```python
from build123d import *

# Parameters (mm, degrees)
SKETCH_1_W          = 60
SKETCH_1_H          = 95
EXTRUDE_1_DEPTH     = 5
SKETCH_2_R          = 1.5
SKETCH_2_R_2        = 1.25
CUT_EXTRUDE_1_DEPTH = 5
FILLET_1_R          = 5
CUT_EXTRUDE_4_DEPTH = 5
FILLET_4_R          = 0.5
FILLET_5_R          = 0.5


with BuildPart() as part:
    # 草图1 → 凸台-拉伸1 (new body)
    with BuildSketch(Plane(origin=(0, 0, 0), x_dir=(1, 0, 0), z_dir=(0, 1, 0))):
        Rectangle(SKETCH_1_W, SKETCH_1_H)
    extrude(amount=EXTRUDE_1_DEPTH)

    # 草图2 → 切除-拉伸1 (cut)
    with BuildSketch(Plane(origin=(0, 5, 0), x_dir=(1, 0, 0), z_dir=(0, 1, 0))):
        with Locations(Location((-24.605, 43.54, 0), (0, 0, 270))):
            Circle(SKETCH_2_R)
        with Locations(Location((24.605, 43.54, 0), (0, 0, 90))):
            Circle(SKETCH_2_R)
        with Locations(Location((24.605, -43.54, 0), (0, 0, 270))):
            Circle(SKETCH_2_R)
        with Locations(Location((-24.605, -43.54, 0), (0, 0, 90))):
            Circle(SKETCH_2_R)
        with Locations(Location((-24.5, 29, 0), (0, 0, 270))):
            Circle(SKETCH_2_R_2)
        with Locations(Location((24.5, 29, 0), (0, 0, 90))):
            Circle(SKETCH_2_R_2)
        with Locations(Location((24.5, -29, 0), (0, 0, 270))):
            Circle(SKETCH_2_R_2)
        with Locations(Location((-24.5, -29, 0), (0, 0, 90))):
            Circle(SKETCH_2_R_2)
    extrude(amount=-CUT_EXTRUDE_1_DEPTH, mode=Mode.SUBTRACT)

    # 圆角1
    fillet_1_edges = [part.edges().sort_by_distance(p)[0] for p in [
        (-30, 2.5, -47.5),
        (30, 2.5, -47.5),
        (30, 2.5, 47.5),
        (-30, 2.5, 47.5),
    ]]
    fillet(fillet_1_edges, radius=FILLET_1_R)

    # 草图3 → 切除-拉伸4 (cut)
    with BuildSketch(Plane.XZ):
        with BuildLine():
            Line((-24.572504286, 39.040117332), (-24.530690396, 33.249889187))
            ThreePointArc((-24.530690396, 33.249889187), (-22.391619047, 32.69015308), (-20.823217786, 31.131612664))
            Line((-20.823217786, 31.131612664), (-3.522175136, 36.25445474))
            Line((-3.522175136, 36.25445474), (-17.995469496, 40.54))
            Line((-17.995469496, 40.54), (-21.250898034, 40.54))
            ThreePointArc((-21.250898034, 40.54), (-22.753062375, 39.438740799), (-24.572504286, 39.040117332))
        make_face()
        with BuildLine():
            Line((-17.775077424, 42.560575343), (0, 37.297371479))
            Line((0, 37.297371479), (17.775077424, 42.560575343))
            ThreePointArc((17.775077424, 42.560575343), (18.12794912, 43.111720539), (17.63311969, 43.54))
            Line((17.63311969, 43.54), (-17.63311969, 43.54))
            ThreePointArc((-17.63311969, 43.54), (-18.12794912, 43.111720539), (-17.775077424, 42.560575343))
        make_face()
        with BuildLine():
            ThreePointArc((-22.264395713, 25.385505088), (-23.33791209, 24.911962367), (-24.5, 24.75))
            Line((-24.5, 24.75), (-24.5, -24.75))
            ThreePointArc((-24.5, -24.75), (-23.522899134, -24.863845518), (-22.598145824, -25.199282871))
            Line((-22.598145824, -25.199282871), (-1.176126043, 0.157393604))
            Line((-1.176126043, 0.157393604), (-22.264395713, 25.385505088))
        make_face()
        with BuildLine():
            Line((20.255386851, 29.213914036), (0, 35.211538001))
            Line((0, 35.211538001), (-20.255386851, 29.213914036))
            ThreePointArc((-20.255386851, 29.213914036), (-20.376517668, 27.970731589), (-20.853820398, 26.816453731))
            Line((-20.853820398, 26.816453731), (0.134149451, 1.708331943))
            Line((0.134149451, 1.708331943), (21.070374573, 26.48998617))
            ThreePointArc((21.070374573, 26.48998617), (20.428338154, 27.781775959), (20.255386851, 29.213914036))
        make_face()
        with BuildLine():
            Line((21.250898034, 40.54), (17.995469496, 40.54))
            Line((17.995469496, 40.54), (3.522175136, 36.25445474))
            Line((3.522175136, 36.25445474), (20.823217786, 31.131612664))
            ThreePointArc((20.823217786, 31.131612664), (22.391619047, 32.69015308), (24.530690396, 33.249889187))
            Line((24.530690396, 33.249889187), (24.572504286, 39.040117332))
            ThreePointArc((24.572504286, 39.040117332), (22.753062375, 39.438740799), (21.250898034, 40.54))
        make_face()
        with BuildLine():
            Line((-24.530690396, -33.249889187), (-24.572504286, -39.040117332))
            ThreePointArc((-24.572504286, -39.040117332), (-22.753062375, -39.438740799), (-21.250898034, -40.54))
            Line((-21.250898034, -40.54), (-17.995469496, -40.54))
            Line((-17.995469496, -40.54), (-3.522175136, -36.25445474))
            Line((-3.522175136, -36.25445474), (-20.823217786, -31.131612664))
            ThreePointArc((-20.823217786, -31.131612664), (-22.391619047, -32.69015308), (-24.530690396, -33.249889187))
        make_face()
        with BuildLine():
            Line((24.5, -24.75), (24.5, 24.75))
            ThreePointArc((24.5, 24.75), (23.522899134, 24.863845518), (22.598145824, 25.199282871))
            Line((22.598145824, 25.199282871), (1.436295206, 0.150561732))
            Line((1.436295206, 0.150561732), (22.618050588, -25.189387659))
            ThreePointArc((22.618050588, -25.189387659), (23.533719101, -24.861304405), (24.5, -24.75))
        make_face()
        with BuildLine():
            Line((0.126019713, -1.400376607), (-21.070374573, -26.48998617))
            ThreePointArc((-21.070374573, -26.48998617), (-20.428338154, -27.781775959), (-20.255386851, -29.213914036))
            Line((-20.255386851, -29.213914036), (0, -35.211538001))
            Line((0, -35.211538001), (20.255386851, -29.213914036))
            ThreePointArc((20.255386851, -29.213914036), (20.431537904, -27.771132157), (21.083549516, -26.472082658))
            Line((21.083549516, -26.472082658), (0.126019713, -1.400376607))
        make_face()
        with BuildLine():
            Line((17.775077424, -42.560575343), (0, -37.297371479))
            Line((0, -37.297371479), (-17.775077424, -42.560575343))
            ThreePointArc((-17.775077424, -42.560575343), (-18.12794912, -43.111720539), (-17.63311969, -43.54))
            Line((-17.63311969, -43.54), (17.63311969, -43.54))
            ThreePointArc((17.63311969, -43.54), (18.12794912, -43.111720539), (17.775077424, -42.560575343))
        make_face()
        with BuildLine():
            Line((3.522175136, -36.25445474), (17.995469496, -40.54))
            Line((17.995469496, -40.54), (21.250898034, -40.54))
            ThreePointArc((21.250898034, -40.54), (22.753062375, -39.438740799), (24.572504286, -39.040117332))
            Line((24.572504286, -39.040117332), (24.530690396, -33.249889187))
            ThreePointArc((24.530690396, -33.249889187), (22.391619047, -32.69015308), (20.823217786, -31.131612664))
            Line((20.823217786, -31.131612664), (3.522175136, -36.25445474))
        make_face()
    extrude(amount=-CUT_EXTRUDE_4_DEPTH, mode=Mode.SUBTRACT)

    # 圆角4
    fillet_4_edges = [part.edges().sort_by_distance(p)[0] for p in [
        (-20.823217786, 2.5, 31.131612664),
        (-24.530690396, 2.5, 33.249889187),
        (-24.572504286, 2.5, 39.040117332),
        (-21.250898034, 2.5, 40.54),
        (-3.522175136, 2.5, 36.25445474),
        (-21.250898034, 2.5, -40.54),
        (-24.572504286, 2.5, -39.040117332),
        (-24.530690396, 2.5, -33.249889187),
        (-20.823217786, 2.5, -31.131612664),
        (-3.522175136, 2.5, -36.25445474),
        (-20.853820398, 2.5, 26.816453731),
        (-20.255386851, 2.5, 29.213914036),
        (-20.255386851, 2.5, -29.213914036),
        (-21.070374573, 2.5, -26.48998617),
        (-22.264395713, 2.5, 25.385505088),
        (-1.176126043, 2.5, 0.157393604),
        (-22.598145824, 2.5, -25.199282871),
        (-24.5, 2.5, -24.75),
        (-24.5, 2.5, 24.75),
    ]]
    fillet(fillet_4_edges, radius=FILLET_4_R)

    # 圆角5
    fillet_5_edges = [part.edges().sort_by_distance(p)[0] for p in [
        (24.530690396, 2.5, 33.249889187),
        (20.823217786, 2.5, 31.131612664),
        (21.250898034, 2.5, 40.54),
        (24.572504286, 2.5, 39.040117332),
        (1.436295206, 2.5, 0.150561732),
        (22.598145824, 2.5, 25.199282871),
        (24.5, 2.5, 24.75),
        (24.5, 2.5, -24.75),
        (22.618050588, 2.5, -25.189387659),
        (20.255386851, 2.5, 29.213914036),
        (21.070374573, 2.5, 26.48998617),
        (0.134149451, 2.5, 1.708331943),
        (21.083549516, 2.5, -26.472082658),
        (20.255386851, 2.5, -29.213914036),
        (0.126019713, 2.5, -1.400376607),
        (24.572504286, 2.5, -39.040117332),
        (21.250898034, 2.5, -40.54),
        (3.522175136, 2.5, -36.25445474),
        (20.823217786, 2.5, -31.131612664),
        (24.530690396, 2.5, -33.249889187),
    ]]
    fillet(fillet_5_edges, radius=FILLET_5_R)


solid = part.part
```
For this review, take the finished solid that the model builds, in its own axes (mm). Round coordinates to 2 decimals unless told otherwise and drop trailing zeros. Answer as CSV lines item,"result". Start each with the question number.
(1) For line 1 (X direction, y = 2.5, z = -29); line 2 (X direction, y = 1.5, z = -17); line 3 (Z direction, x = -1.5, y = 2.5), list the stretches that pass through material, from the lowest coordinate up.
(2) Mouldability with a two-part tool opening along X and no side actions: class faces 1 (the cylindrical face through (-20.43, 2.46, -27.77)), 2 (the cylindrical face through (-28.57, 2.54, 46)) as +X half, -X half, draft (parallel to the pull), parting line (faces both ways), or undercut.
(3) For pin 1 (1.8 mm diameter, centred on x = -24.605, z = 43.54, fed in from -Y), flat-tipped, find the tip position at first contact; note if it passes through.
(4) Add section A-A, the plane x = -8. State how many separate pieces and enclosed holes the cut face has, plus the area to 3 significant figures.
From the geometry:
1,line 1,"x = -30 to -25.75, -23.25 to -20.23, 20.23 to 23.25, 25.75 to 30"
1,line 2,"x = -30 to -24.5, -15.67 to -13.05, 13.17 to 15.77, 24.5 to 30"
1,line 3,"z = -47.5 to -43.54, -37.74 to -34.77, -3.33 to -0.23, 0.54 to 3.66, 34.77 to 37.74, 43.54 to 47.5"
2,face 1,"undercut"
2,face 2,"-X half"
3,pin 1,"passes through"
4,separate pieces,"8"
4,enclosed holes,"0"
4,area,"112 mm²"
